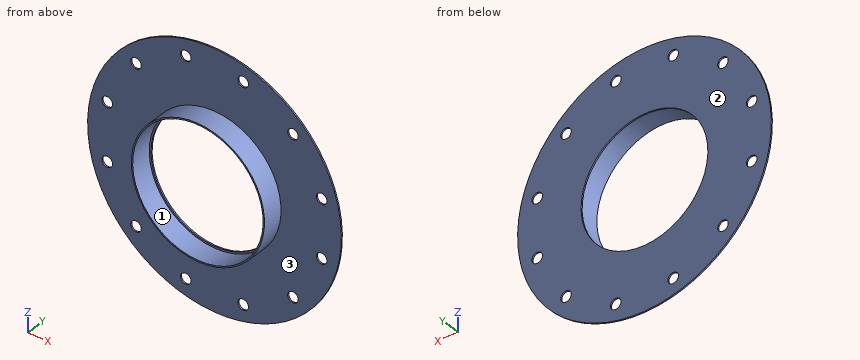
from build123d import *

# Parameters (mm, degrees)
BOSS_EXTRUDE1_DEPTH     = 6.35
CUT_EXTRUDE1_DEPTH      = 849.551897352
CUT_EXTRUDE1_DEPTH_BACK = 849.551897352
SKETCH2_R               = 25
SKETCH3_R               = 315
SKETCH3_R_2             = 308.65
BOSS_EXTRUDE2_DEPTH     = 100


with BuildPart() as part:
    # Sketch1 → Boss-Extrude1 (new body)
    with BuildSketch(Plane(origin=(0, 0, 0), x_dir=(1, 0, 0), z_dir=(0, 1, 0))):
        with BuildLine():
            Line((0, 450), (0, 300))
            ThreePointArc((0, 300), (212.132034356, 212.132034356), (300, 0))
            ThreePointArc((300, 0), (212.132034356, -212.132034356), (0, -300))
            Line((0, -300), (0, -450))
            ThreePointArc((0, -450), (318.198051534, -318.198051534), (450, 0))
            ThreePointArc((450, 0), (318.198051534, 318.198051534), (0, 450))
        make_face()
        with BuildLine():
            ThreePointArc((0, -450), (-450, 0), (0, 450))
            Line((0, 450), (0, 600))
            ThreePointArc((0, 600), (-600, 0), (0, -600))
            Line((0, -600), (0, -450))
        make_face()
        with BuildLine():
            Line((0, 600), (0, 450))
            ThreePointArc((0, 450), (318.198051534, 318.198051534), (450, 0))
            ThreePointArc((450, 0), (318.198051534, -318.198051534), (0, -450))
            Line((0, -450), (0, -600))
            ThreePointArc((0, -600), (424.264068712, -424.264068712), (600, 0))
            ThreePointArc((600, 0), (424.264068712, 424.264068712), (0, 600))
        make_face()
        with BuildLine():
            ThreePointArc((0, -300), (-300, 0), (0, 300))
            Line((0, 300), (0, 450))
            ThreePointArc((0, 450), (-450, 0), (0, -450))
            Line((0, -450), (0, -300))
        make_face()
    extrude(amount=BOSS_EXTRUDE1_DEPTH)

    # Sketch2 → Cut-Extrude1 (cut, two sides: drawn at the far end of the back side and taken through both)
    with BuildSketch(Plane(origin=(0, 6.35, 0), x_dir=(1, 0, 0), z_dir=(0, 1, 0)).offset(-CUT_EXTRUDE1_DEPTH_BACK)):
        with Locations(Location((135.879998679, 507.111058802, 0), (0, 0, 270))):
            Circle(SKETCH2_R)
        with Locations(Location((-135.879998679, 507.111058802, 0), (0, 0, 270))):
            Circle(SKETCH2_R)
        with Locations(Location((371.231060123, 371.231060123, 0), (0, 0, 270))):
            Circle(SKETCH2_R)
        with Locations(Location((507.111058802, 135.879998679, 0), (0, 0, 270))):
            Circle(SKETCH2_R)
        with Locations(Location((507.111058802, -135.879998679, 0), (0, 0, 270))):
            Circle(SKETCH2_R)
        with Locations(Location((371.231060123, -371.231060123, 0), (0, 0, 270))):
            Circle(SKETCH2_R)
        with Locations(Location((135.879998679, -507.111058802, 0), (0, 0, 270))):
            Circle(SKETCH2_R)
        with Locations(Location((-371.231060123, 371.231060123, 0), (0, 0, 270))):
            Circle(SKETCH2_R)
        with Locations(Location((-507.111058802, 135.879998679, 0), (0, 0, 270))):
            Circle(SKETCH2_R)
        with Locations(Location((-507.111058802, -135.879998679, 0), (0, 0, 270))):
            Circle(SKETCH2_R)
        with Locations(Location((-371.231060123, -371.231060123, 0), (0, 0, 270))):
            Circle(SKETCH2_R)
        with Locations(Location((-135.879998679, -507.111058802, 0), (0, 0, 270))):
            Circle(SKETCH2_R)
    extrude(amount=CUT_EXTRUDE1_DEPTH + CUT_EXTRUDE1_DEPTH_BACK, mode=Mode.SUBTRACT)

    # Sketch3 → Boss-Extrude2 (add)
    with BuildSketch(Plane.XZ):
        with Locations(Location((0, 0, 0), (0, 0, 90))):
            Circle(SKETCH3_R)
        with Locations(Location((0, 0, 0), (0, 0, 270))):
            Circle(SKETCH3_R_2, mode=Mode.SUBTRACT)
    extrude(amount=BOSS_EXTRUDE2_DEPTH)


solid = part.part
The listing builds one solid part. Answer for the finished solid, in the listing's coordinates (mm). Face numbers are marked on the shaded views. Give positions to 0.01 mm unless a question says otherwise; leave off trailing zeros. Write each loop counter-clockwise with the first axis right and the second up, starting at its lowest first coordinate (ties: lowest second). Pieces come first, ordered by that corner, then holes.
Item 1: Section B-B, the plane x = 0 is taken. Write down the section's boundary in (y, z), plus the area to 3 significant figures.
Item 2: Flat-ended cylindrical pins translate along their axes: P1, Ø5, axis at y = -56, z = 23, coming from the +X side; P2, Ø12, axis at x = -198.5, y = -23.5, coming from the -Z side; P3, Ø12, axis at x = 46, y = -71, coming from the -Z side. Find the tip coordinate at first contact, or state that the pin passes through.
Item 3: Determine the mould class of the marked faces 1, 2 and 3 for opening direction Y: released by +Y, released by -Y, zero draft, split by the parting line, or undercut.
Item 4: Section A-A, the plane z = 0 is taken. Write down the section's boundary in (x, y), plus the area to 3 significant figures.
Item 5: Section C-C, the plane y = -61 is taken. Write down the section's boundary in (x, z), plus the area to 3 significant figures.
Item 6: Section D-D, the plane x = 466 is taken. Write down the section's boundary in (y, z), plus the area to 3 significant figures.
Item 7: Find the intervals of material crossed by line 1 along Z through (x, y) = (3.5, -86); line 2 along Y through (x, z) = (299.5, 474); line 3 along Z through (x, y) = (-245.5, -38), in increasing order.
Completed:
1. outline: (-100, -315) - (0, -315) - (0, -600) - (6.35, -600) - (6.35, -300) - (0, -300) - (0, -308.65) - (-100, -308.65) - close; (-100, 308.65) - (0, 308.65) - (0, 300) - (6.35, 300) - (6.35, 600) - (0, 600) - (0, 315) - (-100, 315) - close
1. area: 5,080 mm2
2. P1: stops at x = 314.33
2. P2: stops at z = -249.34
2. P3: stops at z = -312.45
3. face 1: zero draft
3. face 2: released by +Y
3. face 3: released by -Y
4. outline: (-600, 0) - (-315, 0) - (-315, -100) - (-308.65, -100) - (-308.65, 0) - (-300, 0) - (-300, 6.35) - (-600, 6.35) - close; (300, 0) - (308.65, 0) - (308.65, -100) - (315, -100) - (315, 0) - (600, 0) - (600, 6.35) - (300, 6.35) - close
4. area: 5,080 mm2
5. outline: circle Ø630 at (0, 0); hole circle Ø617.3 at (0, 0)
5. area: 12,400 mm2
6. outline: (0, -377.95) - (6.35, -377.95) - (6.35, 377.95) - (0, 377.95) - close
6. area: 4,800 mm2
7. line 1: z = -314.98 to -308.63, 308.63 to 314.98
7. line 2: y = 0 to 6.35
7. line 3: z = -197.37 to -187.07, 187.07 to 197.37
